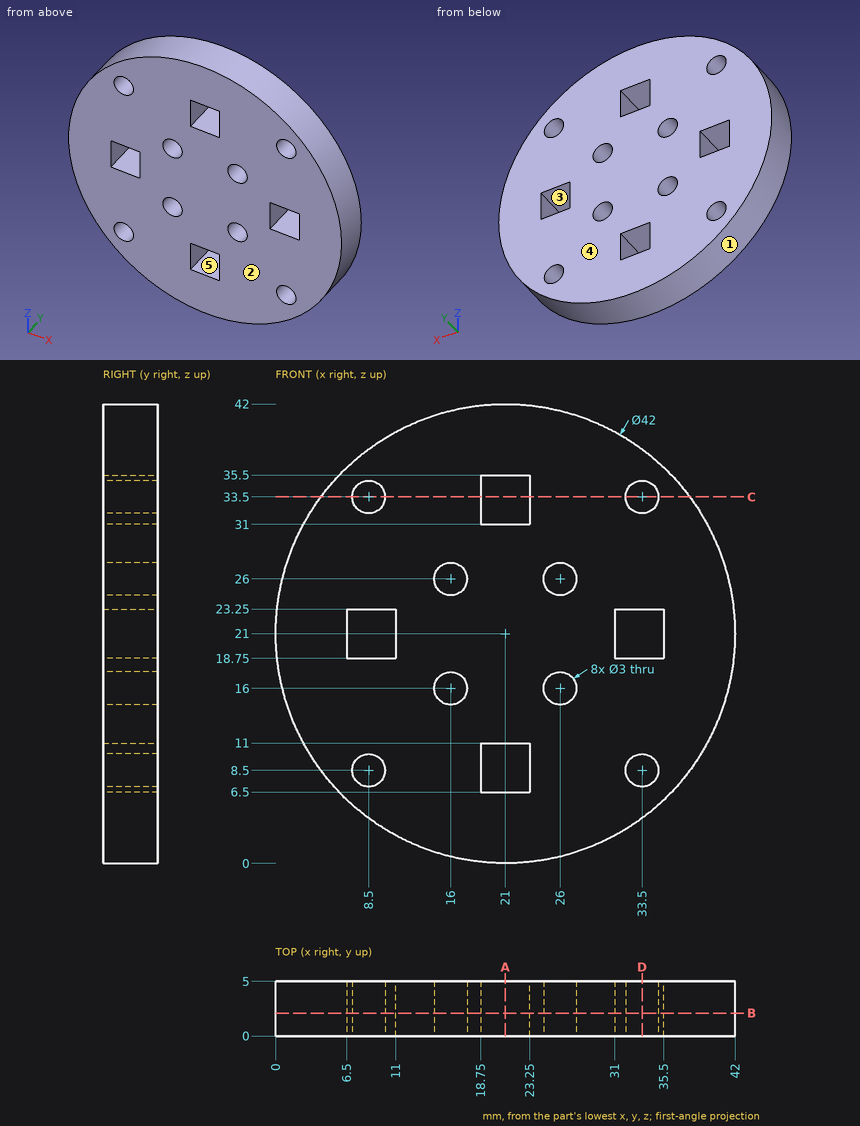
Input: dimensioned drawing with shaded views. Units: mm. Origin: part minimum x, y, z. A direction names the side the tool comes from. Give positions to 0.01 mm unless a question says otherwise; leave off trailing zeros. Order: outer loops, then holes, each group sorted by start corner. A loop starts at its lowest first (then second) coordinate and runs counter-clockwise, first axis right, second up. Notation, with made-up numbers: (11.25, 56.25) -> (15.25, 56.25) arc R31 cw to (15.25, 95.25) -> close; hole circle Ø10 at (-26, 39.5). An arc over 180 degrees is marked (long way). Answer as a JSON object with one key per item and string values.
Q1. Access query for the marked faces 4 and 5. Directions: +Z, -Z, +X, -X, +Y, -Y. A direction counts if a zero-diameter tool reaches every point of the face in a straight line with its end or side. Return the directions, or none.
Entries:
{"face 4": "+Z, -Z, +X, -X, +Y", "face 5": "+Y, -Y"}
Q2. Section A-A (x = 21). Output: boundary loops of the cut face in (y, z), plus the area to 3 significant figures.
Entries:
{"outline": "(0, 0) -> (5, 0) -> (5, 6.5) -> (0, 6.5) -> close; (0, 11) -> (5, 11) -> (5, 31) -> (0, 31) -> close; (0, 35.5) -> (5, 35.5) -> (5, 42) -> (0, 42) -> close", "area": "165 mm^2"}
Q3. Draft query along Z for the marked faces 1, 2 and 3. Return one class per face: released by +Z, released by -Z, zero draft, split by the parting line, or undercut.
Entries:
{"face 1": "split by the parting line", "face 2": "zero draft", "face 3": "undercut"}
Q4. Section C-C (z = 33.5). Output: boundary loops of the cut face in (x, y), plus the area to 3 significant figures.
Entries:
{"outline": "(4.13, 0) -> (7, 0) -> (7, 5) -> (4.13, 5) -> close; (10, 0) -> (18.75, 0) -> (18.75, 5) -> (10, 5) -> close; (23.25, 0) -> (32, 0) -> (32, 5) -> (23.25, 5) -> close; (35, 0) -> (37.87, 0) -> (37.87, 5) -> (35, 5) -> close", "area": "116 mm^2"}
Q5. Section B-B (y = 2.1). State how many separate pieces and enclosed holes the cut face has, plus the area to 3 significant figures.
Entries:
{"separate pieces": "1", "enclosed holes": "12", "area": "1,250 mm^2"}
Q6. First-contact query: pin 1 (12 mm diameter, centred on x = 33.5, z = 20, fed in from -Y); pin 2 (1.3 mm diameter, centred on x = 22, y = 3.5, fed in from +Z); pin 3 (1 mm diameter, centred on x = 35, y = 1.5, fed in from +Z); pin 4 (2 mm diameter, centred on y = 0.5, z = 8, fed in from +X). Flat tips, straight axial feed; report the tip coordinate or a pass-through.
Entries:
{"pin 1": "stops at y = 0", "pin 2": "stops at z = 42", "pin 3": "stops at z = 37.09", "pin 4": "stops at x = 38.23"}
Q7. Section D-D (x = 33.5). Output: boundary loops of the cut face in (y, z).
Entries:
{"outline": "(0, 4.13) -> (5, 4.13) -> (5, 7) -> (0, 7) -> close; (0, 10) -> (5, 10) -> (5, 18.75) -> (0, 18.75) -> close; (0, 23.25) -> (5, 23.25) -> (5, 32) -> (0, 32) -> close; (0, 35) -> (5, 35) -> (5, 37.87) -> (0, 37.87) -> close"}
Q8. Material intervals for probe 1 along Z at (x, y) = (20.5, 4.55); probe 2 along X at (y, z) = (1.25, 26), sorted ascending.
Entries:
{"probe 1": "z = 0.01 to 6.5, 11 to 31, 35.5 to 41.99", "probe 2": "x = 0.6 to 14.5, 17.5 to 24.5, 27.5 to 41.4"}
